Read the model definition and answer for the solid it produces. Units are mm, in the model's axes. Face numbers are marked on the shaded views. A direction names the side the tool comes from. Coordinates: 2 decimals unless noted, no trailing zeros. Write each loop counter-clockwise with the first axis right and the second up, starting at its lowest first coordinate (ties: lowest second). Pieces come first, ordered by that corner, then holes. Notation, with made-up numbers: (-3.5, 26) -> (3.5, 26) arc R15 cw to (3.5, 32) -> close; hole circle Ø8 at (21, 4.5). An arc over 180 degrees is marked (long way). One line per item, written item: value. Start each with the question number.
1. Given P1, Ø1, axis at x = -24, z = 1.5, coming from the -Y side; P2, Ø4, axis at x = -7, z = -4, coming from the -Y side, each flat-ended and moving along its own axis, determine where each tip first touches the part or whether it passes through.
2. For the marked faces 1 and 2, determine the directions among +Z, -Z, +X, -X, +Y, -Y from which every point of the face is accessible in a straight line to the end or side of a thin tool.
3. Find section A-A, the plane y = 37. Write down the section's boundary in (x, z).
4. Consider line 1 along Y through (x, z) = (-13, -6.25); line 2 along Y through (x, z) = (-14.25, -7.25); line 3 along Z through (x, y) = (-20, 36). Determine where each line is inside the solid, lowest interval first.
5. For a pull along Y with two mould halves and no side action, classify the marked faces 3, 4 and 5 as pulls with the +Y half, pulls with the -Y half, needs draft (parallel to the pull), parting line crosses it, or undercut.
6. Find section C-C, the plane x = -8.25. Write down the section's boundary in (y, z).
7. Find section D-D, the plane y = 17.5. Write down the section's boundary in (x, z).
8. Find section B-B, the plane z = -6.5. Write down the section's boundary in (x, y), and give its area (3 significant figures).
```python
from build123d import *
from build123d.topology import SkipClean

# Parameters (mm, degrees)
SKETCH3_R           = 5
SKETCH3_R_2         = 8
BOSS_EXTRUDE1_DEPTH = 5
BOSS_EXTRUDE4_START = 5
SKETCH4_R           = 8
BOSS_EXTRUDE4_DEPTH = 5
BOSS_EXTRUDE5_START = 5
SKETCH5_R           = 8
SKETCH5_R_2         = 5
BOSS_EXTRUDE5_DEPTH = 5


with BuildPart() as part:
    # Sketch3 → Boss-Extrude1 (new body)
    with BuildSketch(Plane.XY):
        with BuildLine():
            Line((-29.334087167, 80.795829607), (-29.334087167, 20.795829607))
            ThreePointArc((-29.334087167, 20.795829607), (-14.334087167, 5.795829607), (0.665912833, 20.795829607))
            Line((0.665912833, 20.795829607), (0.665912833, 80.795829607))
            ThreePointArc((0.665912833, 80.795829607), (-14.334087167, 95.795829607), (-29.334087167, 80.795829607))
        make_face()
        with Locations((-14.334087167, 20.795829607)):
            Circle(SKETCH3_R, mode=Mode.SUBTRACT)
        with Locations((-14.334087167, 80.795829607)):
            Circle(SKETCH3_R_2, mode=Mode.SUBTRACT)
    extrude(amount=BOSS_EXTRUDE1_DEPTH)

    # Sketch4 → Boss-Extrude4 (add)
    with SkipClean():  # the faces are left unmerged after this step: merging them gives an invalid solid
        with BuildSketch(Plane(origin=(0, 0, 0), x_dir=(-1, 0, 0), z_dir=(0, 0, -1)).offset(BOSS_EXTRUDE4_START)):
            with BuildLine():
                Line((29.334087167, 80.795829607), (29.334087167, 40.795829607))
                Line((29.334087167, 40.795829607), (-0.665912833, 40.795829607))
                Line((-0.665912833, 40.795829607), (-0.665912833, 80.795829607))
                ThreePointArc((-0.665912833, 80.795829607), (14.334087167, 95.795829607), (29.334087167, 80.795829607))
            make_face()
            with Locations((14.334087167, 80.795829607)):
                Circle(SKETCH4_R, mode=Mode.SUBTRACT)
        extrude(amount=-BOSS_EXTRUDE4_DEPTH)

    # Sketch5 → Boss-Extrude5 (add)
    with SkipClean():  # the faces are left unmerged after this step: merging them gives an invalid solid
        with BuildSketch(Plane(origin=(0, 0, -5), x_dir=(-1, 0, 0), z_dir=(0, 0, -1)).offset(BOSS_EXTRUDE5_START)):
            with BuildLine():
                Line((29.334087167, 20.795829607), (29.334087167, 80.795829607))
                ThreePointArc((29.334087167, 80.795829607), (14.334087167, 95.795829607), (-0.665912833, 80.795829607))
                Line((-0.665912833, 80.795829607), (-0.665912833, 20.795829607))
                ThreePointArc((-0.665912833, 20.795829607), (14.334087167, 5.795829607), (29.334087167, 20.795829607))
            make_face()
            with Locations((14.334087167, 80.795829607)):
                Circle(SKETCH5_R, mode=Mode.SUBTRACT)
            with Locations(Location((14.334087167, 20.795829607, 0), (0, 0, 180))):
                Circle(SKETCH5_R_2, mode=Mode.SUBTRACT)
        extrude(amount=-BOSS_EXTRUDE5_DEPTH)


solid = part.part
```
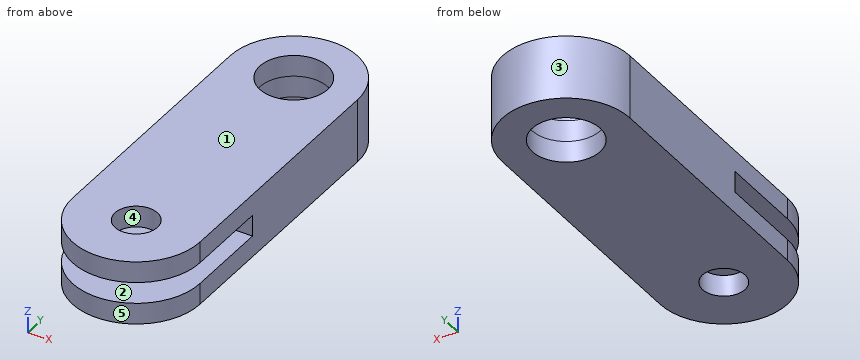
Answer block:
1. P1: stops at y = 8.92
1. P2: stops at y = 6.88
2. face 1: +Z, +X, -X, +Y, -Y
2. face 2: +X, -X, -Y
3. outline: (-29.33, -10) -> (0.67, -10) -> (0.67, -5) -> (-29.33, -5) -> close; (-29.33, 0) -> (0.67, 0) -> (0.67, 5) -> (-29.33, 5) -> close
4. line 1: y = 5.86 to 15.98, 25.61 to 72.91, 88.68 to 95.74
4. line 2: y = 5.8 to 15.8, 25.8 to 72.8, 88.8 to 95.8
4. line 3: z = -10 to -5, 0 to 5
5. face 3: pulls with the +Y half
5. face 4: undercut
5. face 5: pulls with the -Y half
6. outline: (7.09, -10) -> (75.6, -10) -> (75.6, 5) -> (7.09, 5) -> (7.09, 0) -> (40.8, 0) -> (40.8, -5) -> (7.09, -5) -> close; (85.99, -10) -> (94.51, -10) -> (94.51, 5) -> (85.99, 5) -> close
7. outline: (-28.97, -10) -> (-18.09, -10) -> (-18.09, -5) -> (-28.97, -5) -> close; (-28.97, 0) -> (-18.09, 0) -> (-18.09, 5) -> (-28.97, 5) -> close; (-10.57, -10) -> (0.3, -10) -> (0.3, -5) -> (-10.57, -5) -> close; (-10.57, 0) -> (0.3, 0) -> (0.3, 5) -> (-10.57, 5) -> close
8. outline: (-29.33, 20.8) arc R15 ccw to (0.67, 20.8) -> (0.67, 80.8) arc R15 ccw to (-29.33, 80.8) -> close; hole circle Ø16 at (-14.33, 80.8); hole circle Ø10 at (-14.33, 20.8)
8. area: 2,230 mm2
